For this review, take the finished solid that the model builds, in its own axes (mm). Coordinates: 2 decimals unless noted, no trailing zeros. Order: outer loops, then holes, each group sorted by start corner. A loop starts at its lowest first (then second) coordinate and runs counter-clockwise, first axis right, second up. Notation, with made-up numbers: (-38.5, -12) -> (-18.5, -12) arc R16 ccw to (-18.5, -2) -> close; hole circle Ø8 at (38, 35.5). An arc over 180 degrees is marked (long way). Answer as a JSON object with one key per item and string values. Group by question number.
1) Add section C-C, the plane z = 3.4. Write out the cut boundary in (x, y), then the cut area to 3 significant figures.
2) Add section B-B, the plane x = -114.5. Write out the cut boundary in (y, z), then the cut area to 3 significant figures.
3) Wall thickness on L1, parallel to Y at x = -114.5, z = 0.75; L2, parallel to X at y = -24, z = 1.2; L3, parallel to Y at x = -78, z = 2.35: over which ranges is each line inside the solid? List them lowest first.
4) Add section A-A, the plane y = 31. Write out the cut boundary in (x, z).
5) For pin 1 (3.5 mm diameter, centred on x = 114.5, y = -24, fed in from +Z), flat-tipped, find the tip position at first contact; note if it passes through.
6) Draft analysis for pull direction X (two halves, no side actions). For faces 1 (the cylindrical face through (-122.5, 38.9, 1)), 2 (the conical face through (112.12, 31.31, 1.7)), 3 (the flat face through (-2, 1, 4)), 4 (the conical face through (-115.22, 28.71, 1.7)), state which applies: +X half, -X half, draft (parallel to the pull), parting line (faces both ways), or undercut.
from build123d import *

# Parameters (mm, degrees)
ESQUISSE1_W                                 = 249
ESQUISSE1_H                                 = 82
BOSS_EXTRU_1_DEPTH                          = 4
FRAISAGE_POUR_VIS_T_TE_FRAIS_E_M42_AT_COUNT = 2
FRAISAGE_POUR_VIS_T_TE_FRAIS_E_M42_AT_PITCH = 55
FRAISAGE_POUR_VIS_T_TE_FRAIS_E_M42_2_COUNT  = 2
FRAISAGE_POUR_VIS_T_TE_FRAIS_E_M42_2_PITCH  = 229
FRAISAGE_POUR_VIS_T_TE_FRAIS_E_M42_3_COUNT  = 2
FRAISAGE_POUR_VIS_T_TE_FRAIS_E_M42_3_PITCH  = 235.512207752
CONG_1_R                                    = 7
CONG_2_R                                    = 2


with BuildPart() as part:
    # Esquisse1 → Boss.-Extru.1 (new body)
    with BuildSketch(Plane.XY):
        Rectangle(ESQUISSE1_W, ESQUISSE1_H)
    extrude(amount=BOSS_EXTRU_1_DEPTH)

    # Esquisse6 → Fraisage pour vis à tête fraisée M42 (revolve, cut)
    with BuildSketch(Plane(origin=(-114.5, -24, 4), x_dir=(0, -1, 0), z_dir=(1, 0, 0))):
        Polygon((0, 0), (0, 4), (2.25, 4), (2.25, 2.45), (4.7, 0), align=None)
    fraisage_pour_vis_t_te_frais_e_m42 = revolve(axis=Axis((-114.5, -24, 10.35), (0, 0, -1)), mode=Mode.SUBTRACT)

    # Fraisage pour vis à tête fraisée M42 at: Fraisage pour vis à tête fraisée M42 ×2
    with Locations(*[(0, i * FRAISAGE_POUR_VIS_T_TE_FRAIS_E_M42_AT_PITCH, 0) for i in range(1, FRAISAGE_POUR_VIS_T_TE_FRAIS_E_M42_AT_COUNT)]):
        add(fraisage_pour_vis_t_te_frais_e_m42, mode=Mode.SUBTRACT)

    # Fraisage pour vis _ t_te frais_e M42 2: Fraisage pour vis à tête fraisée M42 ×2
    with Locations(*[(i * FRAISAGE_POUR_VIS_T_TE_FRAIS_E_M42_2_PITCH, 0, 0) for i in range(1, FRAISAGE_POUR_VIS_T_TE_FRAIS_E_M42_2_COUNT)]):
        add(fraisage_pour_vis_t_te_frais_e_m42, mode=Mode.SUBTRACT)

    # Fraisage pour vis _ t_te frais_e M42 3: Fraisage pour vis à tête fraisée M42 ×2
    with Locations(*[Vector(0.972348747, 0.233533542, 0) * (i * FRAISAGE_POUR_VIS_T_TE_FRAIS_E_M42_3_PITCH) for i in range(1, FRAISAGE_POUR_VIS_T_TE_FRAIS_E_M42_3_COUNT)]):
        add(fraisage_pour_vis_t_te_frais_e_m42, mode=Mode.SUBTRACT)

    # Congé1
    cong_1_edges = [part.edges().sort_by_distance(p)[0] for p in [
        (124.5, 41, 2),
        (124.5, -41, 2),
        (-124.5, -41, 2),
        (-124.5, 41, 2),
    ]]
    fillet(cong_1_edges, radius=CONG_1_R)

    # Congé2
    cong_2_edges = [part.edges().sort_by_distance(p)[0] for p in [
        (0, 41, 4),
        (124.5, 0, 4),
        (-124.5, 0, 4),
        (0, -41, 4),
        (-122.449747468, 38.949747468, 4),
        (-122.449747468, -38.949747468, 4),
        (122.449747468, -38.949747468, 4),
        (122.449747468, 38.949747468, 4),
    ]]
    fillet(cong_2_edges, radius=CONG_2_R)


solid = part.part
Output values:
{
 "1": {"outline": "(-123.93, -34) arc R6.43 ccw to (-117.5, -40.43) -> (117.5, -40.43) arc R6.43 ccw to (123.93, -34) -> (123.93, 34) arc R6.43 ccw to (117.5, 40.43) -> (-117.5, 40.43) arc R6.43 ccw to (-123.93, 34) -> close; hole circle Ø8.2 at (-114.5, -24); hole circle Ø8.2 at (-114.5, 31); hole circle Ø8.2 at (114.5, -24); hole circle Ø8.2 at (114.5, 31)", "area": "19,800 mm²"},
 "2": {"outline": "(-41, 0) -> (-26.25, 0) -> (-26.25, 1.55) -> (-28.7, 4) -> (-39, 4) arc R2 ccw to (-41, 2) -> close; (-21.75, 0) -> (28.75, 0) -> (28.75, 1.55) -> (26.3, 4) -> (-19.3, 4) -> (-21.75, 1.55) -> close; (33.25, 0) -> (41, 0) -> (41, 2) arc R2 ccw to (39, 4) -> (35.7, 4) -> (33.25, 1.55) -> close", "area": "278 mm²"},
 "3": {"L1": "y = -41 to -26.25, -21.75 to 28.75, 33.25 to 41", "L2": "x = -124.5 to -116.75, -112.25 to 112.25, 116.75 to 124.5", "L3": "y = -40.97 to 40.97"},
 "4": {"outline": "(-124.5, 0) -> (-116.75, 0) -> (-116.75, 1.55) -> (-119.2, 4) -> (-122.5, 4) arc R2 ccw to (-124.5, 2) -> close; (-112.25, 0) -> (112.25, 0) -> (112.25, 1.55) -> (109.8, 4) -> (-109.8, 4) -> (-112.25, 1.55) -> close; (116.75, 0) -> (124.5, 0) -> (124.5, 2) arc R2 ccw to (122.5, 4) -> (119.2, 4) -> (116.75, 1.55) -> close"},
 "5": {"pin 1": "passes through"},
 "6": {"face 1": "-X half", "face 2": "undercut", "face 3": "draft", "face 4": "undercut"}
}
